Geometry: final body of the model. Coordinates: model frame, mm. Round coordinates to 2 decimals unless told otherwise and drop trailing zeros. Write each loop counter-clockwise with the first axis right and the second up, starting at its lowest first coordinate (ties: lowest second). Pieces come first, ordered by that corner, then holes. Notation, with made-up numbers: M 88.25,14 L 121.25,14 A28 cw 121.25,50 Z; hole C 73,37.25 d3. An arc over 180 degrees is marked long. Put each result on its own line as item: value. Start each with the question number.
```python
from build123d import *

# Parameters (mm, degrees)
F0_W     = 50.8
F0_H     = 30.48
F1_DEPTH = 7.62
F2_R     = 3.96875
F3_DEPTH = 25.4


with BuildPart() as f1:
    # F0 (on Top) → F1 (new body)
    with BuildSketch(Plane.XY):
        Rectangle(F0_W, F0_H)
    extrude(amount=F1_DEPTH)

    # F2 (on face) → F3 (cut)
    with BuildSketch(Plane.XY.offset(7.62)):
        with BuildLine():
            ThreePointArc((-20.8661, 0), (-16.89735, -3.96875), (-12.9286, 0))
            ThreePointArc((-12.9286, 0), (-16.89735, 3.96875), (-20.8661, 0))
        make_face()
        with Locations((16.89735, 0)):
            Circle(F2_R)
    extrude(amount=-F3_DEPTH, mode=Mode.SUBTRACT)


solid = f1.part
```
1) Ray query, probe 1 along X at (y, z) = (-0.5, 7.5); probe 2 along Y at (x, z) = (15, 5.25); probe 3 along Y at (x, z) = (-20, 7.25). Return the intervals inside material, ascending.
2) Section A-A, the plane y = 0. Output: boundary loops of the cut face in (x, z), and give its area (3 significant figures).
3) Section C-C, the plane x = -16. Output: boundary loops of the cut face in (y, z), and give its area (3 significant figures).
4) Section B-B, the plane z = 2. Output: boundary loops of the cut face in (x, y).
5) Draft query along Y for faces 1 (the face through (-25.4, 0, 4)), 2 (the face through (0, -15.24, 4)), 3 (the face through (-13.23, -1.52, 3.86)). Return one class per face: +Y half, -Y half, draft (parallel to the pull), parting line (faces both ways), or undercut.
6) First-contact query: pin 1 (5 mm diameter, centred on x = 16.9, y = 0, fed in from -Z). Flat tip, straight axial feed; report the tip coordinate or a pass-through.
Solved:
1. probe 1: x = -25.4 to -20.83, -12.96 to 12.96, 20.83 to 25.4
1. probe 2: y = -15.24 to -3.49, 3.49 to 15.24
1. probe 3: y = -15.24 to -2.47, 2.47 to 15.24
2. outline: M -25.4,0 L -20.87,0 L -20.87,7.62 L -25.4,7.62 Z; M -12.93,0 L 12.93,0 L 12.93,7.62 L -12.93,7.62 Z; M 20.87,0 L 25.4,0 L 25.4,7.62 L 20.87,7.62 Z
2. area: 266 mm2
3. outline: M -15.24,0 L -3.87,0 L -3.87,7.62 L -15.24,7.62 Z; M 3.87,0 L 15.24,0 L 15.24,7.62 L 3.87,7.62 Z
3. area: 173 mm2
4. outline: M -25.4,-15.24 L 25.4,-15.24 L 25.4,15.24 L -25.4,15.24 Z; hole C -16.9,0 d7.94; hole C 16.9,0 d7.94
5. face 1: draft
5. face 2: -Y half
5. face 3: undercut
6. pin 1: passes through
